Verification items for this drawing (mm, ordinates from the low corner). A direction names the side the tool comes from. Round coordinates to 2 decimals unless told otherwise and drop trailing zeros. Loops run counter-clockwise (first coordinate to the right, second up) from the corner with the lowest first, then second, coordinate; pieces in that order, holes last. Notation, with made-up numbers: M -11,17 L 4,17 A17 ccw 4,34 Z; hole C -16,11.25 d9. An arc over 180 degrees is marked long. Write item = value, one per line. Start each with the question number.
(1) Cross-section at D-D on z = 87.5. Record the boundary of the cut face in (x, y).
(2) Go/stop test with a flat-tipped pin: P1, Ø4, axis at x = 16, z = 102.5, coming from the +Y side. Record where the tip stops, or that it passes through.
(3) Cross-section at A-A on y = 21. Record the boundary of the cut face in (x, z), plus the area to 3 significant figures.
(4) Mould release check, pull along X, two halves, no side actions. Record for the marked faces 3, 4, 5 and 6: pulls with the +X half, pulls with the -X half, needs draft (parallel to the pull), parting line crosses it, or undercut.
(5) Cross-section at B-B on y = 54. Record the boundary of the cut face in (x, z), plus the area to 3 significant figures.
(6) Scan lines: L1, parallel to X at y = 55, z = 36; L2, parallel to Z at x = 62, y = 23.5; L3, parallel to Y at x = 49, z = 84.5. Record each from-to range of solid material in increasing order. Write a range as from..to.
(7) Set-up check for the marked faces 1 and 2: record each of +Z, -Z, +X, -X, +Y, -Y from which the full face is reachable in a straight line by a thin tool's end or side.
(8) Cross-section at C-C on x = 35. Record the boundary of the cut face in (y, z).
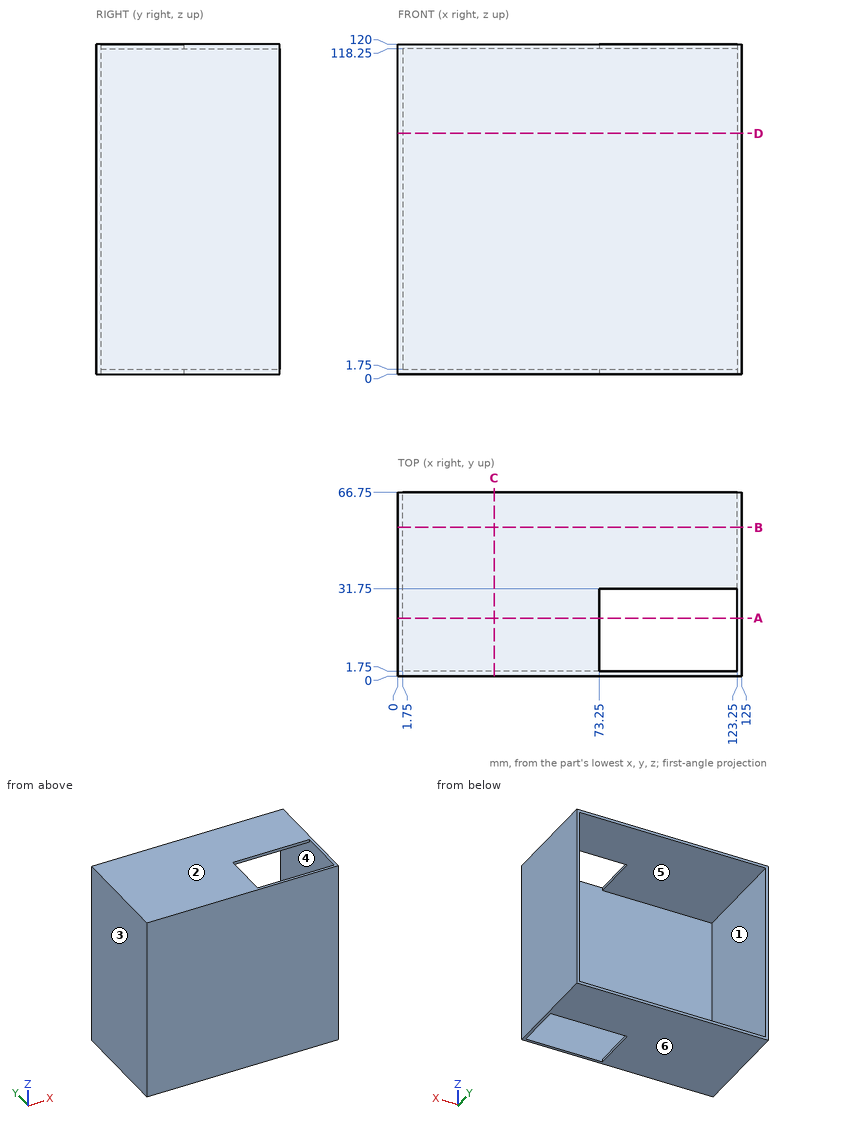
Result:
q1.outline = M 0,0 L 125,0 L 125,66.75 L 123.25,66.75 L 123.25,1.75 L 1.75,1.75 L 1.75,66.75 L 0,66.75 Z
q2.P1 = 1.75
q3.outline = M 0,0 L 73.25,0 L 73.25,1.75 L 1.75,1.75 L 1.75,118.25 L 73.25,118.25 L 73.25,120 L 0,120 Z; M 123.25,0 L 125,0 L 125,120 L 123.25,120 Z
q3.area = 670 mm^2
q4.face_3 = pulls with the -X half
q4.face_4 = undercut
q4.face_5 = undercut
q4.face_6 = needs draft
q5.outline = M 0,0 L 125,0 L 125,120 L 0,120 Z; hole M 1.75,1.75 L 123.25,1.75 L 123.25,118.25 L 1.75,118.25 Z
q5.area = 845 mm^2
q6.L1 = 0..1.75, 123.25..125
q6.L2 = 0..1.75, 118.25..120
q6.L3 = 0..1.75
q7.face_1 = +Y
q7.face_2 = +Z, +X, -X, +Y, -Y
q8.outline = M 0,0 L 66.75,0 L 66.75,1.75 L 1.75,1.75 L 1.75,118.25 L 66.75,118.25 L 66.75,120 L 0,120 Z
